Geometry check sheet. Reference: the model listing, model coordinates, mm. Face numbers are marked on the shaded views. A direction names the side the tool comes from. Give positions to 0.01 mm unless a question says otherwise; leave off trailing zeros. Loops run counter-clockwise (first coordinate to the right, second up) from the corner with the lowest first, then second, coordinate; pieces in that order, holes last. Notation, with made-up numbers: (-32, 30.5) -> (5, 30.5) arc R31 cw to (5, 63.5) -> close; hole circle Ø2 at (15.25, 57). An arc over 180 degrees is marked (long way). Write item = value, one per line.
```python
from build123d import *

# Parameters (mm, degrees)
F0_W     = 45.24375
F0_H     = 45.24375
F0_W_2   = 26.19375
F0_H_2   = 26.19375
F1_DEPTH = 9.525
F0_W_3   = 7.14375
F0_H_3   = 7.14375
F2_DEPTH = 19.05
F3_DEPTH = 6.35


# Not quite as in the source:
# - a length typed as a fraction of an inch, garbled in the dataset ("3 / 203.2 mm" for 3/8 in), is restored


with BuildPart() as f1:
    # F0 (on Top) → F1 (new body)
    with BuildSketch(Plane.XY):
        Rectangle(F0_W, F0_H)
        Rectangle(F0_W_2, F0_H_2, mode=Mode.SUBTRACT)
    extrude(amount=F1_DEPTH)

    # F0 (on Top) → F2 (join)
    with BuildSketch(Plane.XY):
        Rectangle(F0_W_2, F0_H_2)
        Rectangle(F0_W_3, F0_H_3, mode=Mode.SUBTRACT)
    extrude(amount=F2_DEPTH)

    # F0 (on Top) → F3 (join)
    with BuildSketch(Plane.XY):
        Rectangle(F0_W_3, F0_H_3)
    extrude(amount=F3_DEPTH)


solid = f1.part
```
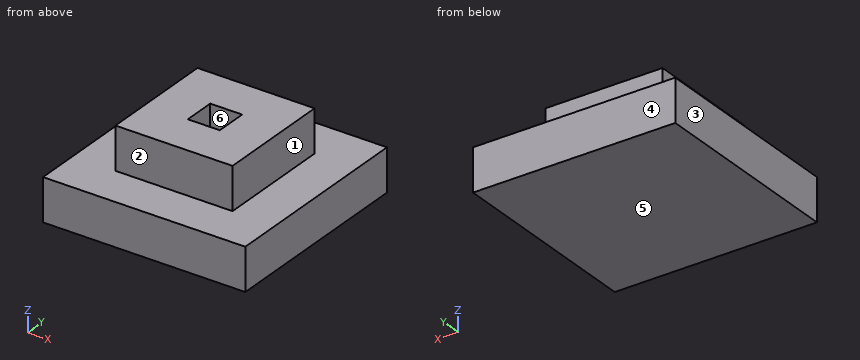
Item 1: Section check B-B, the plane y = -0.5. Record the cut outline in (x, z) (3 decimals).
Answer:
outline = (-22.622, 0) -> (22.622, 0) -> (22.622, 9.525) -> (13.097, 9.525) -> (13.097, 19.05) -> (3.572, 19.05) -> (3.572, 6.35) -> (-3.572, 6.35) -> (-3.572, 19.05) -> (-13.097, 19.05) -> (-13.097, 9.525) -> (-22.622, 9.525) -> close
Item 2: Draft check along Y on the marked faces 4, 5 and 6. Enter one of: +Y half, -Y half, draft (parallel to the pull), parting line (faces both ways), or undercut.
Answer:
face_4 = +Y half
face_5 = draft
face_6 = undercut
Item 3: Thickness scan on L1, parallel to Y at x = 3, z = 10.5; L2, parallel to X at y = -3, z = 8.5. Record the ranges inside material, lowest first. Write a range as [from, to].
Answer:
L1 = [-13.1, -3.57], [3.57, 13.1]
L2 = [-22.62, -3.57], [3.57, 22.62]
Item 4: Section check D-D, the plane z = 12. Record the cut outline in (x, y), plus the area to 3 significant figures.
Answer:
outline = (-13.1, -13.1) -> (13.1, -13.1) -> (13.1, 13.1) -> (-13.1, 13.1) -> close; hole (-3.57, -3.57) -> (3.57, -3.57) -> (3.57, 3.57) -> (-3.57, 3.57) -> close
area = 635 mm^2
Item 5: Tool access check on the marked faces 1, 2 and 3. Record the directions out of +Z, -Z, +X, -X, +Y, -Y that give a thin tool (end or side, any length) a straight path to the whole face; none if there is none.
Answer:
face_1 = +Z, +X, +Y, -Y
face_2 = +Z, +X, -X, -Y
face_3 = +Z, -Z, -X, +Y, -Y
Item 6: Section check A-A, the plane z = 7.75. Record the cut outline in (x, y), plus the area to 3 significant figures.
Answer:
outline = (-22.62, -22.62) -> (22.62, -22.62) -> (22.62, 22.62) -> (-22.62, 22.62) -> close; hole (-3.57, -3.57) -> (3.57, -3.57) -> (3.57, 3.57) -> (-3.57, 3.57) -> close
area = 2,000 mm^2
Item 7: Gauge pin test, flat ends, axial feed: pin 1 (8 mm diameter, centred on x = -0.5, z = 15, fed in from -Y); pin 2 (3 mm diameter, centred on x = 14, z = 16.5, fed in from +Y); pin 3 (5 mm diameter, centred on y = -0.5, z = 14.5, fed in from -X). Record the tip position at first contact, or that the pin passes through.
Answer:
pin_1 = -13.1
pin_2 = 13.1
pin_3 = -13.1
Item 8: Section check C-C, the plane x = -12. Record the cut outline in (y, z) (3 decimals), plus the area to 3 significant figures.
Answer:
outline = (-22.622, 0) -> (22.622, 0) -> (22.622, 9.525) -> (13.097, 9.525) -> (13.097, 19.05) -> (-13.097, 19.05) -> (-13.097, 9.525) -> (-22.622, 9.525) -> close
area = 680 mm^2
